Can you work these out from the model? Positions are in its coordinate system, mm. Face numbers are marked on the shaded views. A direction names the side the tool comes from. Coordinates: 2 decimals unless noted, no trailing zeros. Order: outer loops, then holes, each group sorted by start corner. A loop starts at its lowest first (then second) coordinate and runs counter-clockwise, first axis right, second up. Notation, with made-up numbers: (-19.5, 22) -> (-9.5, 22) arc R28 cw to (-9.5, 46) -> close; hole circle Ø3 at (-3, -27.75). An arc over 180 degrees is marked (long way). Answer as a JSON object with one key per item and string values. Group by question number.
(1) For pin 1 (24.5 mm diameter, centred on y = 0, z = 46.55, fed in from +X); pin 2 (6 mm diameter, centred on x = -16.5, z = 65, fed in from -Y); pin 3 (1.9 mm diameter, centred on x = 3, y = -43, fed in from +Z), each with a flat end and sliding along its axis, tell me the tip position at first contact or that it passes through.
(2) If we mould it in two halves opening along X, with no side actions, what happens to the marked faces 1, 2, 3 and 4? For each: pulls with the +X half, pulls with the -X half, needs draft (parallel to the pull), parting line crosses it, or undercut.
(3) I want a section at B-B, the plane z = 27.5. List the corners of the cut face in (x, y) for me.
(4) I want a section at C-C, the plane y = 0. List the corners of the cut face in (x, z) for me, plus the area to 3 significant figures.
(5) I want a section at D-D, the plane z = 64.5. List the corners of the cut face in (x, y) for me, plus the area to 3 significant figures.
(6) I want a section at A-A, the plane x = 44.5. List the corners of the cut face in (y, z) for me, plus the area to 3 significant figures.
(7) Which directions (+Z, -Z, +X, -X, +Y, -Y) give clear straight access to the entire face, cutting with the end or side of a thin tool? Please do the marked faces 5 and 6.
(8) I need wall thicknesses on line 1 (Y direction, x = -8.5, z = 46); line 2 (Z direction, x = 68, y = 0); line 3 (X direction, y = 22.5, z = 25). Which ranges of each line are inside material? Lowest first, please.
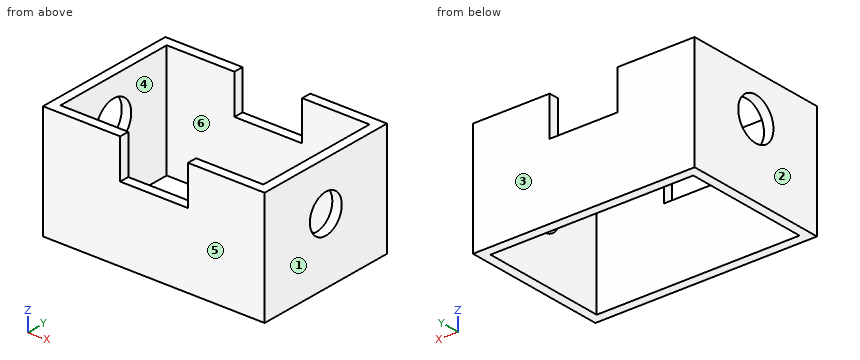
from build123d import *

# Parameters (mm, degrees)
F0_W      = 142.8750008345
F0_H      = 94.9427485466
F0_W_2    = 130.7075917721
F0_H_2    = 82.4066177011
F1_DEPTH  = 47.752
F3_DEPTH  = 25.4
F5_DEPTH  = 25.4
F7_R      = 12.3686155683
F8_DEPTH  = 25.4
F9_R      = 13.6525334008
F10_DEPTH = 25.4


with BuildPart() as f1:
    # F0 (on Top) → F1 (new body)
    with BuildSketch(Plane.XY):
        Rectangle(F0_W, F0_H)
        Rectangle(F0_W_2, F0_H_2, mode=Mode.SUBTRACT)
    extrude(amount=F1_DEPTH)

    # F2 (on face) → F3 (join)
    with BuildSketch(Plane.XY.offset(47.752)):
        Polygon((71.4375004172, -47.4713742733), (71.4375004172, 47.4713742733), (22.0016445965, 47.4713742733), (22.0016445965, 41.2033088505), (65.353795886, 41.2033088505), (65.353795886, -41.2033088505), (22.0016445965, -41.2033088505), (22.0016445965, -47.4713742733), align=None)
    extrude(amount=F3_DEPTH)

    # F4 (on face) → F5 (join)
    with BuildSketch(Plane.XY.offset(47.752)):
        Polygon((-21.6760756448, 47.4713742733), (-71.4375004172, 47.4713742733), (-71.4375004172, -47.4713742733), (-21.6760756448, -47.4713742733), (-21.6760756448, -41.2033088505), (-65.353795886, -41.2033088505), (-65.353795886, 41.2033088505), (-21.6760756448, 41.2033088505), align=None)
    extrude(amount=F5_DEPTH)

    # F7 (on face) → F8 (cut)
    with BuildSketch(Plane.YZ.offset(71.4375004172)):
        with Locations((0, 41.9407263398)):
            Circle(F7_R)
    extrude(amount=-F8_DEPTH, mode=Mode.SUBTRACT)

    # F9 (on face) → F10 (cut)
    with BuildSketch(Plane(origin=(-71.4375004172, 0, 0), x_dir=(0, -1, 0), z_dir=(-1, 0, 0))):
        with Locations((0, 46.5495996177)):
            Circle(F9_R)
    extrude(amount=-F10_DEPTH, mode=Mode.SUBTRACT)


solid = f1.part
Computed values:
{
 "1": {"pin 1": "stops at x = 71.44", "pin 2": "passes through", "pin 3": "stops at z = 47.75"},
 "2": {"face 1": "pulls with the +X half", "face 2": "pulls with the -X half", "face 3": "needs draft", "face 4": "undercut"},
 "3": {"outline": "(-71.44, -47.47) -> (71.44, -47.47) -> (71.44, 47.47) -> (-71.44, 47.47) -> close; hole (-65.35, -41.2) -> (65.35, -41.2) -> (65.35, 41.2) -> (-65.35, 41.2) -> close"},
 "4": {"outline": "(-71.44, 0) -> (-65.35, 0) -> (-65.35, 32.9) -> (-71.44, 32.9) -> close; (-71.44, 60.2) -> (-65.35, 60.2) -> (-65.35, 73.15) -> (-71.44, 73.15) -> close; (65.35, 0) -> (71.44, 0) -> (71.44, 29.57) -> (65.35, 29.57) -> close; (65.35, 54.31) -> (71.44, 54.31) -> (71.44, 73.15) -> (65.35, 73.15) -> close", "area": "573 mm2"},
 "5": {"outline": "(-71.44, -47.47) -> (-21.68, -47.47) -> (-21.68, -41.2) -> (-65.35, -41.2) -> (-65.35, 41.2) -> (-21.68, 41.2) -> (-21.68, 47.47) -> (-71.44, 47.47) -> close; (22, -47.47) -> (71.44, -47.47) -> (71.44, 47.47) -> (22, 47.47) -> (22, 41.2) -> (65.35, 41.2) -> (65.35, -41.2) -> (22, -41.2) -> close", "area": "2,250 mm2"},
 "6": {"outline": "(-47.47, 0) -> (-41.2, 0) -> (-41.2, 73.15) -> (-47.47, 73.15) -> close; (41.2, 0) -> (47.47, 0) -> (47.47, 73.15) -> (41.2, 73.15) -> close", "area": "917 mm2"},
 "7": {"face 5": "+Z, -Z, +X, -X, -Y", "face 6": "+Z, -Z"},
 "8": {"line 1": "y = -47.47 to -41.2, 41.2 to 47.47", "line 2": "z = 0 to 29.57, 54.31 to 73.15", "line 3": "x = -71.44 to -65.35, 65.35 to 71.44"}
}
